Can you work these out from the model? Positions are in its coordinate system, mm. Face numbers are marked on the shaded views. A direction names the side the tool comes from. Round coordinates to 2 decimals unless told otherwise and drop trailing zeros. Loops run counter-clockwise (first coordinate to the right, second up) from the corner with the lowest first, then second, coordinate; pieces in that order, holes last.
(1) Which directions (+Z, -Z, +X, -X, +Y, -Y) give clear straight access to the entire face, cutting with the end or side of a thin tool? Please do the marked faces 1 and 2.
(2) Thinking about a two-plate mould opening in X: for the marked faces 3, 4 and 5, which applies, released by +X, released by -X, zero draft, split by the parting line, or undercut?
(3) I want a section at D-D on z = 10.75. Write out the boundary of the cut face in (x, y), plus the area to 3 significant figures.
(4) Will these pins go through, and if not, where does the flat tip stop? pin 1 Ø3 at (x, z) = (28, 5) entering from -Y; pin 2 Ø2 at (x, y) = (18, 13.5) entering from +Z.
(5) I want a section at A-A on z = 6. Write out the boundary of the cut face in (x, y).
(6) I want a section at B-B on x = 23.5. Write out the boundary of the cut face in (y, z).
(7) If I drill on line 1 along Y through (x, z) = (37, 8); line 2 along X through (y, z) = (18.5, 3.5); line 3 along Z through (x, y) = (32, 23.5), over which ranges is the centre line in solid material (lowest first)?
(8) I want a section at C-C on y = 12. Write out the boundary of the cut face in (x, z).
from build123d import *

# Parameters (mm, degrees)
F0_W        = 58
F0_H        = 32
F1_DEPTH    = 13
F2_T        = -2
F3_T1_DEPTH = 83


# Not quite as in the source:
# - a fillet or chamfer that OpenCascade refuses, or shapes differently, is made with other operations: its cross-section is extruded or revolved along the edge and cut away or added


with BuildPart() as f1:
    # F0 (on Top) → F1 (new body)
    with BuildSketch(Plane.XY):
        with Locations((29, 16)):
            Rectangle(F0_W, F0_H)
    extrude(amount=F1_DEPTH)

    # F2
    f2_openings = [f1.faces().sort_by_distance(p)[0] for p in [
        (29, 16, 13),
    ]]
    offset(amount=F2_T, openings=f2_openings)

    # F3: fillet of radius 5 on 2 edges, made by hand

    # F3_s2 → F3_t1 (cut)
    with BuildSketch(Plane.YZ.offset(-12.5)):
        with BuildLine():
            ThreePointArc((0, 8), (1.4644660941, 11.5355339059), (5, 13))
            Line((5, 13), (0, 13))
            Line((0, 13), (0, 8))
        make_face()
        with BuildLine():
            ThreePointArc((32, 8), (30.5355339059, 11.5355339059), (27, 13))
            Line((27, 13), (32, 13))
            Line((32, 13), (32, 8))
        make_face()
    extrude(amount=F3_T1_DEPTH, mode=Mode.SUBTRACT)


solid = f1.part
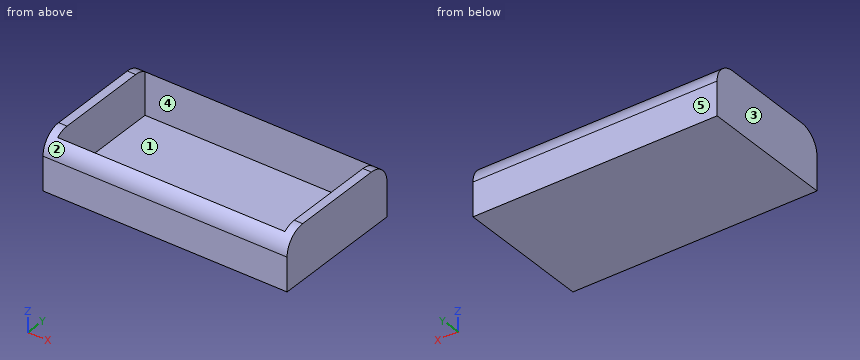
Filled sheet:
1. face 1: +Z
1. face 2: +Z, +X, -X, -Y
2. face 3: released by -X
2. face 4: undercut
2. face 5: zero draft
3. outline: (0, 0.82) - (58, 0.82) - (58, 31.18) - (0, 31.18) - close; hole (2, 2) - (56, 2) - (56, 30) - (2, 30) - close
3. area: 248 mm2
4. pin 1: stops at y = 0
4. pin 2: stops at z = 2
5. outline: (0, 0) - (58, 0) - (58, 32) - (0, 32) - close; hole (2, 2) - (56, 2) - (56, 30) - (2, 30) - close
6. outline: (0, 0) - (32, 0) - (32, 8) arc R5 ccw to (30, 12) - (30, 2) - (2, 2) - (2, 12) arc R5 ccw to (0, 8) - close
7. line 1: y = 0 to 2, 30 to 32
7. line 2: x = 0 to 2, 56 to 58
7. line 3: z = 0 to 2
8. outline: (0, 0) - (58, 0) - (58, 13) - (56, 13) - (56, 2) - (2, 2) - (2, 13) - (0, 13) - close
